Here's how the part is built. I have some questions about the finished solid (model axes, mm). Face numbers are marked on the shaded views. A direction names the side the tool comes from. Coordinates: 2 decimals unless noted, no trailing zeros. Loops run counter-clockwise (first coordinate to the right, second up) from the corner with the lowest first, then second, coordinate; pieces in that order, holes last. Notation, with made-up numbers: (22.5, -17.5) -> (38.5, -17.5) arc R34 cw to (38.5, 16.5) -> close; hole circle Ø7 at (-24, 5.25). An arc over 180 degrees is marked (long way). Answer as a JSON object with one key per item and string values. Group by question number.
Q1. On a 3-axis mill with a long thin cutter (end or side, diameter ignored), from which of +Z, -Z, +X, -X, +Y, -Y can I reach the whole of each face in a straight line? I mean the marked faces 5, 6 and 7. Say none if no direction works.
Q2. I want a section at B-B on x = 8.5. Write out the boundary of the cut face in (y, z).
Q3. I want a section at C-C on z = -19.7. Write out the boundary of the cut face in (x, y).
Q4. Thinking about a two-plate mould opening in X: for the marked faces 1, 2, 3 and 4, which applies, released by +X, released by -X, zero draft, split by the parting line, or undercut?
Q5. I need wall thicknesses on line 1 (X direction, y = 2, z = -56); line 2 (Y direction, x = 28.5, z = -59.7); line 3 (X direction, y = 22.5, z = -5). Which ranges of each line are inside material? Lowest first, please.
Q6. I want a section at A-A on z = -55.9. Write out the boundary of the cut face in (x, y), then the cut area to 3 significant figures.
Q7. I want a section at D-D on z = -41.2. Write out the boundary of the cut face in (x, y), then the cut area to 3 significant figures.
Q8. I'm going to push flat-ended pins straight in: pin 1 (4 mm diameter, centred on x = 61, y = 19, fed in from +Z); pin 2 (2 mm diameter, centred on y = 24.5, z = -3, fed in from +X); pin 3 (2.5 mm diameter, centred on y = 8.56, z = -49.4, fed in from -X); pin 4 (5 mm diameter, centred on x = 57.5, z = -31, fed in from -Y). Where does each tip first touch, or does it pass through?
```python
from build123d import *

# Parameters (mm, degrees)
SKETCH_2_R           = 1.6
SKETCH_2_R_2         = 17
SKETCH_2_R_3         = 1.65
EXTRUDE_2_DEPTH      = 3.5
EXTRUDE_3_DEPTH      = 18
EXTRUDE_4_DEPTH      = 10
CUT_EXTRUDE_5_DEPTH  = 3
SKETCH_10_R          = 2.75
SKETCH_10_R_2        = 1.6
CUT_EXTRUDE_4_DEPTH  = 5
SKETCH_14_R          = 1.55
SKETCH_14_R_2        = 1.1
CUT_EXTRUDE_6_DEPTH  = 10
CUT_EXTRUDE_7_DEPTH  = 2
EXTRUDE_6_DEPTH      = 2
EXTRUDE_7_DEPTH      = 2.5
SKETCH_21_R          = 1.6
SKETCH_21_R_2        = 14
CUT_EXTRUDE_8_DEPTH  = 3
FILLET_1_R           = 1
SKETCH_25_R          = 1.66119801
CUT_EXTRUDE_9_DEPTH  = 10
CUT_EXTRUDE_START    = -10
SKETCH_27_R          = 1.66119801
CUT_EXTRUDE_10_DEPTH = 10


with BuildPart() as part:
    # 草图2 → 凸台-拉伸2 (new body)
    with BuildSketch(Plane(origin=(0, 0, 0), x_dir=(1, 0, 0), z_dir=(0, 1, 0))):
        Polygon((-9, 34.9), (-9, 61), (6, 61), (51, 61), (66, 61), (66, 34.9), (57, 34.9), (57, 0), (0, 0), (0, 34.9), align=None)
        with Locations(Location((21.5, 56, 0), (0, 0, 270))):
            Circle(SKETCH_2_R, mode=Mode.SUBTRACT)
        with Locations(Location((35.5, 56, 0), (0, 0, 270))):
            Circle(SKETCH_2_R, mode=Mode.SUBTRACT)
        with Locations(Location((28.5, 25.7, 0), (0, 0, 270))):
            Circle(SKETCH_2_R_2, mode=Mode.SUBTRACT)
        with Locations(Location((44, 41.2, 0), (0, 0, 270))):
            Circle(SKETCH_2_R_3, mode=Mode.SUBTRACT)
        with Locations(Location((44, 10.2, 0), (0, 0, 270))):
            Circle(SKETCH_2_R_3, mode=Mode.SUBTRACT)
        with Locations(Location((13, 10.2, 0), (0, 0, 270))):
            Circle(SKETCH_2_R_3, mode=Mode.SUBTRACT)
        with Locations(Location((13, 41.2, 0), (0, 0, 270))):
            Circle(SKETCH_2_R_3, mode=Mode.SUBTRACT)
    extrude(amount=EXTRUDE_2_DEPTH)

    # 草图6 → 凸台-拉伸3 (add)
    with BuildSketch(Plane(origin=(0, 3.5, 0), x_dir=(1, 0, 0), z_dir=(0, 1, 0))):
        Polygon((66, 61), (-9, 61), (-9, 34.9), (0, 34.9), (0, 0), (57, 0), (57, 34.9), (66, 34.9), align=None)
        Polygon((15.5, 59), (-7, 59), (-7, 36.9), (2.5, 36.9), (2.5, 4), (54.5, 4), (54.5, 36.9), (64, 36.9), (64, 59), (41.5, 59), align=None, mode=Mode.SUBTRACT)
    extrude(amount=EXTRUDE_3_DEPTH)

    # 草图11 → 凸台-拉伸4 (add)
    with BuildSketch(Plane(origin=(0, 21.5, 0), x_dir=(1, 0, 0), z_dir=(0, 1, 0))):
        Polygon((2.5, 36.9), (2.5, 4), (54.5, 4), (54.5, 36.9), (57, 36.9), (57, 0), (0, 0), (0, 36.9), align=None)
    extrude(amount=EXTRUDE_4_DEPTH)

    # 草图12 → 切除-拉伸5 (cut)
    with BuildSketch(Plane.ZY):
        Polygon((-36.9, 21.5), (-4, 31.5), (-36.9, 31.5), align=None)
    extrude(amount=-CUT_EXTRUDE_5_DEPTH, mode=Mode.SUBTRACT)

    # 草图10 → 切除-拉伸4 (cut)
    with BuildSketch(Plane.XY):
        with Locations((28.5, 17.071067812)):
            Circle(SKETCH_10_R)
        with Locations((35.571067812, 24.142135624)):
            Circle(SKETCH_10_R_2)
        with Locations((35.571067812, 10)):
            Circle(SKETCH_10_R_2)
        with Locations((21.428932188, 10)):
            Circle(SKETCH_10_R_2)
        with Locations((21.428932188, 24.142135624)):
            Circle(SKETCH_10_R_2)
    extrude(amount=-CUT_EXTRUDE_4_DEPTH, mode=Mode.SUBTRACT)

    # 草图14 → 切除-拉伸6 (cut)
    with BuildSketch(Plane(origin=(0, 0, -61), x_dir=(-1, 0, 0), z_dir=(0, 0, -1))):
        with Locations((31.5, 17.071067812)):
            Circle(SKETCH_14_R)
        with Locations((-88.5, 17.071067812)):
            Circle(SKETCH_14_R)
        with Locations((-28.5, 17.071067812)):
            Circle(SKETCH_14_R_2)
        with Locations((-13.5, 17.071067812)):
            Circle(SKETCH_14_R_2)
        with Locations((1.5, 17.071067812)):
            Circle(SKETCH_14_R_2)
        with Locations((-43.5, 17.071067812)):
            Circle(SKETCH_14_R_2)
        with Locations((-58.5, 17.071067812)):
            Circle(SKETCH_14_R_2)
    extrude(amount=-CUT_EXTRUDE_6_DEPTH, mode=Mode.SUBTRACT)

    # 草图20 → 切除-拉伸7 (cut)
    with BuildSketch(Plane(origin=(0, 0, -4), x_dir=(-1, 0, 0), z_dir=(0, 0, -1))):
        Polygon((-24.428932188, 22.410084816), (-21.428932188, 20.678034009), (-18.428932188, 22.410084816), (-18.428932188, 25.874186431), (-21.428932188, 27.606237239), (-24.428932188, 25.874186431), align=None)
        Polygon((-33.839017004, 21.142135624), (-32.106966197, 24.142135624), (-33.839017004, 27.142135624), (-37.303118619, 27.142135624), (-39.035169427, 24.142135624), (-37.303118619, 21.142135624), align=None)
        Polygon((-23.160982996, 13), (-24.893033803, 10), (-23.160982996, 7), (-19.696881381, 7), (-17.964830573, 10), (-19.696881381, 13), align=None)
        Polygon((-32.571067812, 11.732050808), (-35.571067812, 13.464101615), (-38.571067812, 11.732050808), (-38.571067812, 8.267949192), (-35.571067812, 6.535898385), (-32.571067812, 8.267949192), align=None)
    extrude(amount=-CUT_EXTRUDE_7_DEPTH, mode=Mode.SUBTRACT)

    # 草图22 → 凸台-拉伸6 (add)
    with BuildSketch(Plane(origin=(0, 0, -36.9), x_dir=(-1, 0, 0), z_dir=(0, 0, -1))):
        Polygon((-57, 31.5), (-64.002075382, 21.5), (-57, 21.5), align=None)
    extrude(amount=-EXTRUDE_6_DEPTH)

    # 草图24 → 凸台-拉伸7 (add)
    with BuildSketch(Plane(origin=(57, 0, 0), x_dir=(0, 0, -1), z_dir=(1, 0, 0))):
        Polygon((0, 31.5), (3.464101615, 37.5), (33.435898385, 37.5), (36.9, 31.5), align=None)
    extrude(amount=-EXTRUDE_7_DEPTH)

    # 草图21 → 切除-拉伸8 (cut)
    with BuildSketch(Plane(origin=(57, 0, 0), x_dir=(0, 0, -1), z_dir=(1, 0, 0))):
        with Locations((7.7, 33.2)):
            Circle(SKETCH_21_R)
        with Locations((31.7, 33.2)):
            Circle(SKETCH_21_R)
        with Locations((31.7, 9.2)):
            Circle(SKETCH_21_R)
        with Locations((7.7, 9.2)):
            Circle(SKETCH_21_R)
        with Locations((19.7, 21.2)):
            Circle(SKETCH_21_R_2)
    extrude(amount=-CUT_EXTRUDE_8_DEPTH, mode=Mode.SUBTRACT)

    # 圆角1
    fillet_1_edges = [part.edges().sort_by_distance(p)[0] for p in [
        (66, 0, -47.95),
        (61.5, 0, -34.9),
        (57, 0, -17.45),
        (28.5, 0, 0),
        (0, 0, -17.45),
        (-4.5, 0, -34.9),
        (-9, 0, -47.95),
        (66, 10.75, -61),
        (66, 10.75, -34.9),
        (57, 15.75, 0),
        (0, 15.75, 0),
        (0, 10.75, -34.9),
        (-9, 10.75, -34.9),
        (-9, 10.75, -61),
    ]]
    fillet(fillet_1_edges, radius=FILLET_1_R)

    # 草图25 → 切除-拉伸9 (cut)
    with BuildSketch(Plane(origin=(66, 0, 0), x_dir=(0, 0, -1), z_dir=(1, 0, 0))):
        with Locations((55.9, 8.56)):
            Circle(SKETCH_25_R)
        with Locations((49.4, 8.56)):
            Circle(SKETCH_25_R)
    extrude(amount=-CUT_EXTRUDE_9_DEPTH, mode=Mode.SUBTRACT)

    # 草图27 → 切除-拉伸10 (cut)
    with BuildSketch(Plane.ZY.offset(9).offset(CUT_EXTRUDE_START)):
        with Locations(Location((-55.9, 8.56, 0), (0, 0, 180))):
            Circle(SKETCH_27_R)
        with Locations(Location((-49.4, 8.56, 0), (0, 0, 180))):
            Circle(SKETCH_27_R)
    extrude(amount=CUT_EXTRUDE_10_DEPTH, mode=Mode.SUBTRACT)


solid = part.part
```
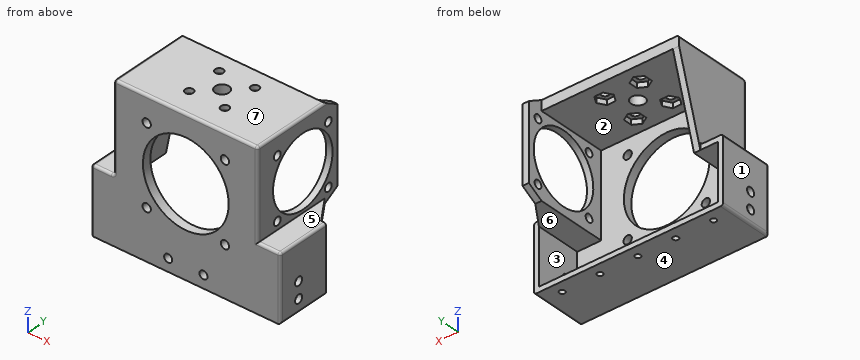
Result set:
{
 "1": {"face 5": "+Z, +X, +Y, -Y", "face 6": "+Y", "face 7": "+Z, +X, -X, +Y, -Y"},
 "2": {"outline": "(0, -61) -> (21.5, -61) -> (21.5, -59) -> (3.5, -59) -> (3.5, -4) -> (31.5, -4) -> (31.5, 0) -> (1, 0) arc R1 ccw to (0, -1) -> close"},
 "3": {"outline": "(0, 1) arc R1 ccw to (1, 0) -> (12.59, 0) -> (12.59, 3.5) -> (2.5, 3.5) -> (2.5, 26.73) -> (0, 26.73) -> close; (44.41, 0) -> (56, 0) arc R1 ccw to (57, 1) -> (57, 7.2) -> (54.5, 7.2) -> (54.5, 3.5) -> (44.41, 3.5) -> close; (54.5, 35.2) -> (57, 35.2) -> (57, 37.5) -> (54.5, 37.5) -> close"},
 "4": {"face 1": "released by -X", "face 2": "undercut", "face 3": "undercut", "face 4": "zero draft"},
 "5": {"line 1": "x = -9 to 19.9, 23.1 to 33.9, 37.1 to 66", "line 2": "y = 0 to 15.97, 18.17 to 21.5", "line 3": "x = 0 to 2.5, 54.5 to 57"},
 "6": {"outline": "(-9, 1) arc R1 ccw to (-8, 0) -> (19.9, 0) -> (19.9, 3.5) -> (-7, 3.5) -> (-7, 6.9) -> (-9, 6.9) -> close; (-9, 10.22) -> (-7, 10.22) -> (-7, 21.5) -> (-9, 21.5) -> close; (23.1, 0) -> (33.9, 0) -> (33.9, 3.5) -> (23.1, 3.5) -> close; (37.1, 0) -> (65, 0) arc R1 ccw to (66, 1) -> (66, 6.9) -> (64, 6.9) -> (64, 3.5) -> (37.1, 3.5) -> close; (64, 10.22) -> (66, 10.22) -> (66, 21.5) -> (64, 21.5) -> close", "area": "298 mm²"},
 "7": {"outline": "(-9, 1) arc R1 ccw to (-8, 0) -> (11.35, 0) -> (11.35, 3.5) -> (-7, 3.5) -> (-7, 21.5) -> (-9, 21.5) -> close; (14.65, 0) -> (21.52, 0) -> (21.52, 3.5) -> (14.65, 3.5) -> close; (35.48, 0) -> (42.35, 0) -> (42.35, 3.5) -> (35.48, 3.5) -> close; (45.65, 0) -> (65, 0) arc R1 ccw to (66, 1) -> (66, 21.5) -> (64, 21.5) -> (64, 3.5) -> (45.65, 3.5) -> close", "area": "262 mm²"},
 "8": {"pin 1": "stops at z = -34.9", "pin 2": "stops at x = 57", "pin 3": "passes through", "pin 4": "stops at y = 0"}
}
